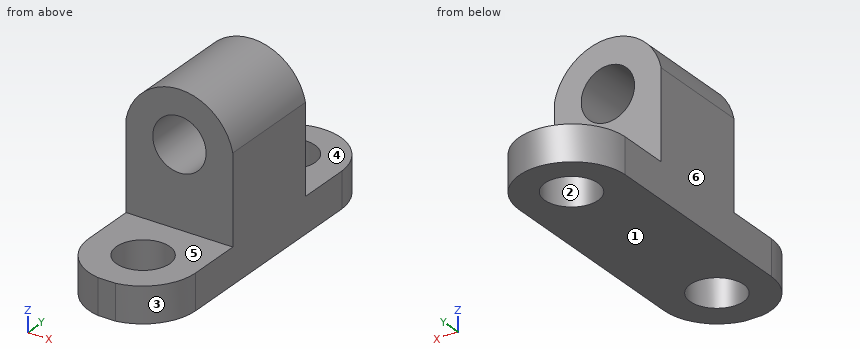
```python
from build123d import *

# Parameters (mm, degrees)
F1_DEPTH  = 25.4
F2_R      = 6.35
F3_DEPTH  = 25.4
F4_R      = 6.35
F5_DEPTH  = 25.4
F7_DEPTH  = 25.4
F9_DEPTH  = 25.4
F11_DEPTH = 25.4


with BuildPart() as f1:
    # F0 (on Right) → F1 (new body)
    with BuildSketch(Plane.YZ):
        Polygon((0, 8.4666666667), (0, 0), (76.2, 0), (76.2, 8.4666666667), (50.8, 8.4666666667), (50.8, 40.2166666667), (25.4, 40.2166666667), (25.4, 8.4666666667), align=None)
    extrude(amount=F1_DEPTH)

    # F2 (on face) → F3 (cut)
    with BuildSketch(Plane(origin=(0, 50.8, 0), x_dir=(-1, 0, 0), z_dir=(0, 1, 0))):
        with Locations((-12.7, 27.5166666667)):
            Circle(F2_R)
    extrude(amount=-F3_DEPTH, mode=Mode.SUBTRACT)

    # F4 (on face) → F5 (cut)
    with BuildSketch(Plane.XY.offset(8.4666666667)):
        with Locations((12.7, 63.5)):
            Circle(F4_R)
        with Locations((12.7, 12.7)):
            Circle(F4_R)
    extrude(amount=-F5_DEPTH, mode=Mode.SUBTRACT)

    # F6 (on face) → F7 (cut)
    with BuildSketch(Plane.XY.offset(8.4666666667)):
        with BuildLine():
            ThreePointArc((0, 63.5), (12.7, 75.8324942144), (25.4, 63.5))
            Line((25.4, 63.5), (25.4, 76.2))
            Line((25.4, 76.2), (0, 76.2))
            Line((0, 76.2), (0, 63.5))
        make_face()
    extrude(amount=-F7_DEPTH, mode=Mode.SUBTRACT)

    # F8 (on face) → F9 (cut)
    with BuildSketch(Plane.XY.offset(8.4666666667)):
        with BuildLine():
            ThreePointArc((10.5819482078, 0), (3.0561269403, 4.2579759584), (0, 12.3467603626))
            Line((0, 12.3467603626), (0, 0))
            Line((0, 0), (10.5819482078, 0))
        make_face()
        with BuildLine():
            ThreePointArc((25.4, 12.3467603626), (22.3438730597, 4.2579759584), (14.8180517922, 0))
            Line((14.8180517922, 0), (25.4, 0))
            Line((25.4, 0), (25.4, 12.3467603626))
        make_face()
    extrude(amount=-F9_DEPTH, mode=Mode.SUBTRACT)

    # F10 (on face) → F11 (cut)
    with BuildSketch(Plane.XZ.offset(-25.4)):
        with BuildLine():
            ThreePointArc((0, 29.4869819596), (12.7, 39.8722781395), (25.4, 29.4869819596))
            Line((25.4, 29.4869819596), (25.4, 40.2166666667))
            Line((25.4, 40.2166666667), (0, 40.2166666667))
            Line((0, 40.2166666667), (0, 29.4869819596))
        make_face()
    extrude(amount=-F11_DEPTH, mode=Mode.SUBTRACT)


solid = f1.part
```
Model file for the job. Use its own axes, mm. Face numbers are marked on the shaded views. A direction names the side the tool comes from. Give positions to 0.01 mm unless a question says otherwise; leave off trailing zeros. Write each loop counter-clockwise with the first axis right and the second up, starting at its lowest first coordinate (ties: lowest second). Pieces come first, ordered by that corner, then holes. Notation, with made-up numbers: (6, 31.5) -> (48, 31.5) arc R28 cw to (48, 55.5) -> close; hole circle Ø7 at (-31, 41). An arc over 180 degrees is marked (long way). Use CSV: the item, a comma, the result in double quotes. Start each with the question number.
1) Tool access for the marked faces 4, 5 and 6: list every direction of +Z, -Z, +X, -X, +Y, -Y with a clear straight run to the whole face (end or side of a thin tool).
2) Cut at C-C on z = 32.5. List the corners of the cut face in (x, y), plus the area to 3 significant figures.
3) Drill centre lines: L1, parallel to Y at x = 12.7, z = 4.75; L2, parallel to Y at x = 19.75, z = 29; L3, parallel to Z at x = 15.75, y = 27.5. Where is each one in solid material? Low to high.
4) Two-plate mould, pull along X, no slides. Class the marked faces 1, 2 and 3: released by +X, released by -X, zero draft, split by the parting line, or undercut.
5) Pin check, flat tips, straight feed: P1, Ø8, axis at y = 37, z = 16.5, coming from the -X side; P2, Ø1, axis at x = 9.5, z = 15, coming from the -Y side; P3, Ø3, axis at x = 16, z = 34, coming from the +Y side; P4, Ø8, axis at x = 18.5, y = 40.5, coming from the +Z side. Stop position of each tip, or through.
6) Cut at A-A on x = 12.7. List the corners of the cut face in (y, z).
7) Cut at B-B on y = 62. List the corners of the cut face in (x, z).
8) Cut at D-D on y = 49.5. List the corners of the cut face in (x, z).
Final values:
1,face 4,"+Z, +X, -X, +Y"
1,face 5,"+Z, +X, -X, -Y"
1,face 6,"+Z, -Z, -X, +Y, -Y"
2,outline,"(1.01, 25.4) -> (8.76, 25.4) -> (8.76, 50.8) -> (1.01, 50.8) -> close; (16.64, 25.4) -> (24.39, 25.4) -> (24.39, 50.8) -> (16.64, 50.8) -> close"
2,area,"394 mm2"
3,L1,"y = 0 to 6.35, 19.05 to 57.15, 69.85 to 75.83"
3,L2,"y = 25.4 to 50.8"
3,L3,"z = 0 to 21.95, 33.09 to 39.51"
4,face 1,"zero draft"
4,face 2,"undercut"
4,face 3,"released by +X"
5,P1,"stops at x = 0"
5,P2,"stops at y = 25.4"
5,P3,"stops at y = 50.8"
5,P4,"stops at z = 39.75"
6,outline,"(0, 0) -> (6.35, 0) -> (6.35, 8.47) -> (0, 8.47) -> close; (19.05, 0) -> (57.15, 0) -> (57.15, 8.47) -> (50.8, 8.47) -> (50.8, 21.17) -> (25.4, 21.17) -> (25.4, 8.47) -> (19.05, 8.47) -> close; (25.4, 33.87) -> (50.8, 33.87) -> (50.8, 39.87) -> (25.4, 39.87) -> close; (69.85, 0) -> (75.83, 0) -> (75.83, 8.47) -> (69.85, 8.47) -> close"
7,outline,"(0, 0) -> (6.53, 0) -> (6.53, 8.47) -> (0, 8.47) -> close; (18.87, 0) -> (25.4, 0) -> (25.4, 8.47) -> (18.87, 8.47) -> close"
8,outline,"(0, 0) -> (25.4, 0) -> (25.4, 29.49) arc R12.96 ccw to (0, 29.49) -> close; hole circle Ø12.7 at (12.7, 27.52)"
